from build123d import *

# Parameters (mm, degrees)
BOSS_EXTRUDE1_DEPTH = 1.524


with BuildPart() as part:
    # Sketch1 → Boss-Extrude1 (new body)
    with BuildSketch(Plane(origin=(0, 0, 0), x_dir=(1, 0, 0), z_dir=(0, 1, 0))):
        with BuildLine():
            Line((5.520593562, 10.562997869), (7.050708645, 17.571208446))
            ThreePointArc((7.050708645, 17.571208446), (7.131145016, 17.829150642), (7.238606677, 18.077054207))
            ThreePointArc((7.238606677, 18.077054207), (7.564510049, 19.45989002), (7.637457251, 20.878736946))
            ThreePointArc((7.637457251, 20.878736946), (8.492098945, 20.073618252), (9.504942938, 19.47966911))
            ThreePointArc((9.504942938, 19.47966911), (10.499295157, 19.276273595), (11.333912028, 18.698761041))
            Line((11.333912028, 18.698761041), (10.277523058, 13.457219083))
            Line((10.277523058, 13.457219083), (11.773700319, 13.155201971))
            Line((11.773700319, 13.155201971), (12.828772876, 18.399768932))
            ThreePointArc((12.828772876, 18.399768932), (13.409499296, 18.538098505), (14.004660893, 18.584584187))
            ThreePointArc((14.004660893, 18.584584187), (16.746835107, 19.097796263), (19.463914435, 19.730556864))
            ThreePointArc((19.463914435, 19.730556864), (18.823035781, 17.184750652), (17.837865312, 14.751379768))
            ThreePointArc((17.837865312, 14.751379768), (17.528924841, 13.243726046), (16.651902084, 11.979093671))
            Line((16.651902084, 11.979093671), (13.544076564, 9.012401066))
            Line((13.544076564, 9.012401066), (14.59914963, 7.908648182))
            Line((14.59914963, 7.908648182), (17.221929817, 10.411217166))
            ThreePointArc((17.221929817, 10.411217166), (19.571015538, 11.015907736), (21.993615768, 10.893995741))
            ThreePointArc((21.993615768, 10.893995741), (20.058776223, 8.670441452), (18.698609679, 6.055533286))
            ThreePointArc((18.698609679, 6.055533286), (16.478620051, 2.831263642), (16.457225541, -1.083300314))
            ThreePointArc((16.457225541, -1.083300314), (16.55614989, -1.524335384), (16.589363804, -1.975106719))
            ThreePointArc((16.589363804, -1.975106719), (16.624442109, -4.753141238), (17.243254302, -7.461605332))
            ThreePointArc((17.243254302, -7.461605332), (15.84253831, -5.968117791), (14.035036599, -5.006115769))
            Line((14.035036599, -5.006115769), (12.161156101, -1.197565278))
            Line((12.161156101, -1.197565278), (10.792144449, -1.871143044))
            Line((10.792144449, -1.871143044), (12.582390495, -5.515217687))
            ThreePointArc((12.582390495, -5.515217687), (12.984657899, -6.771031753), (13.401445653, -8.022101696))
            ThreePointArc((13.401445653, -8.022101696), (10.284977839, -6.689966631), (7.846889336, -4.335676947))
            ThreePointArc((7.846889336, -4.335676947), (6.119650246, -3.528046665), (4.880261331, -4.977024464))
            Line((4.880261331, -4.977024464), (4.878620901, -9.02232865))
            ThreePointArc((4.878620901, -9.02232865), (3.451641907, -14.873313942), (2.99866015, -20.878736946))
            ThreePointArc((2.99866015, -20.878736946), (2.023183201, -17.933730156), (0.761997186, -15.099293685))
            Line((0.761997186, -15.099293685), (0.761997186, -7.081931903))
            Line((0.761997186, -7.081931903), (-0.761997186, -7.081931903))
            Line((-0.761997186, -7.081931903), (-0.761997186, -15.100287099))
            ThreePointArc((-0.761997186, -15.100287099), (-2.023137189, -17.934235169), (-2.99866015, -20.878736946))
            ThreePointArc((-2.99866015, -20.878736946), (-3.451641907, -14.873313942), (-4.878620901, -9.02232865))
            Line((-4.878620901, -9.02232865), (-4.880261331, -4.977024464))
            ThreePointArc((-4.880261331, -4.977024464), (-6.119650246, -3.528046665), (-7.846889336, -4.335676947))
            ThreePointArc((-7.846889336, -4.335676947), (-10.284977839, -6.689966631), (-13.401445653, -8.022101696))
            ThreePointArc((-13.401445653, -8.022101696), (-12.984657899, -6.771031753), (-12.582390495, -5.515217687))
            Line((-12.582390495, -5.515217687), (-10.792144449, -1.871143044))
            Line((-10.792144449, -1.871143044), (-12.161156101, -1.197565278))
            Line((-12.161156101, -1.197565278), (-14.035036599, -5.006115769))
            ThreePointArc((-14.035036599, -5.006115769), (-15.84253831, -5.968117791), (-17.243254302, -7.461605332))
            ThreePointArc((-17.243254302, -7.461605332), (-16.624442109, -4.753141238), (-16.589363804, -1.975106719))
            ThreePointArc((-16.589363804, -1.975106719), (-16.55614989, -1.524335384), (-16.457225541, -1.083300314))
            ThreePointArc((-16.457225541, -1.083300314), (-16.478620051, 2.831263642), (-18.698609679, 6.055533286))
            ThreePointArc((-18.698609679, 6.055533286), (-20.058776223, 8.670441452), (-21.993615768, 10.893995741))
            ThreePointArc((-21.993615768, 10.893995741), (-19.571015538, 11.015907736), (-17.221929817, 10.411217166))
            Line((-17.221929817, 10.411217166), (-14.59914963, 7.908648182))
            Line((-14.59914963, 7.908648182), (-13.544076564, 9.012401066))
            Line((-13.544076564, 9.012401066), (-16.651902084, 11.979093671))
            ThreePointArc((-16.651902084, 11.979093671), (-17.528924841, 13.243726046), (-17.837865312, 14.751379768))
            ThreePointArc((-17.837865312, 14.751379768), (-18.823035781, 17.184750652), (-19.463914435, 19.730556864))
            ThreePointArc((-19.463914435, 19.730556864), (-16.746835107, 19.097796263), (-14.004660893, 18.584584187))
            ThreePointArc((-14.004660893, 18.584584187), (-13.409499296, 18.538098505), (-12.828772876, 18.399768932))
            Line((-12.828772876, 18.399768932), (-11.773700319, 13.155201971))
            Line((-11.773700319, 13.155201971), (-10.277523058, 13.457219083))
            Line((-10.277523058, 13.457219083), (-11.333912028, 18.698761041))
            ThreePointArc((-11.333912028, 18.698761041), (-10.499295157, 19.276273595), (-9.504942938, 19.47966911))
            ThreePointArc((-9.504942938, 19.47966911), (-8.492098945, 20.073618252), (-7.637457251, 20.878736946))
            ThreePointArc((-7.637457251, 20.878736946), (-7.564510049, 19.45989002), (-7.238606677, 18.077054207))
            ThreePointArc((-7.238606677, 18.077054207), (-7.131145016, 17.829150642), (-7.050708645, 17.571208446))
            Line((-7.050708645, 17.571208446), (-5.520593562, 10.562997869))
            ThreePointArc((-5.520593562, 10.562997869), (-3.516439493, 7.545594261), (0.000595641, 6.678517605))
            ThreePointArc((0.000595641, 6.678517605), (3.516886937, 7.546036839), (5.520593562, 10.562997869))
        make_face()
    extrude(amount=BOSS_EXTRUDE1_DEPTH)


solid = part.part
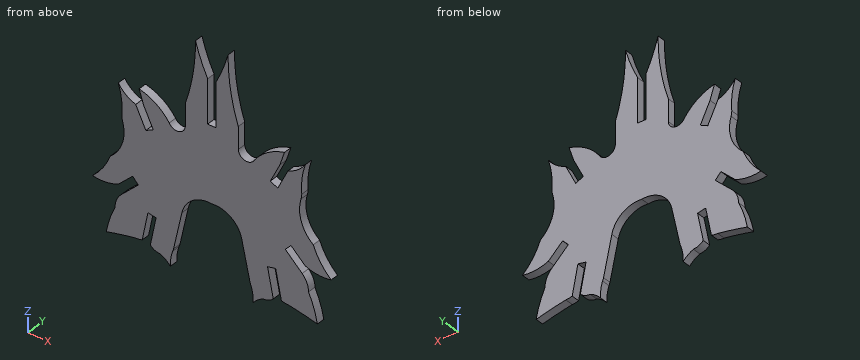
Part model, mm, in its own coordinate system. Coordinates: 2 decimals unless noted, no trailing zeros. Order: outer loops, then holes, each group sorted by start corner. A loop starts at its lowest first (then second) coordinate and runs counter-clockwise, first axis right, second up. Notation, with made-up numbers: M 24.5,-11 L 53.5,-11 A26 ccw 53.5,6 Z; hole C 47,-8 d9. An arc over 180 degrees is marked long. One line per question, with ' | ' between items.
Q1. Slice it at C-C (x = 3.5). Give the cut face in (y, z), and give its area (3 significant figures).
A:
outline: M 0,-7.53 L 1.52,-7.53 L 1.52,14.58 L 0,14.58 Z | area: 33.7 mm^2
Q2. Slice it at A-A (z = -14). Give the cut face in (x, y), and give its area (3 significant figures).
A:
outline: M -17.76,0 L -11.94,0 L -11.94,1.52 L -17.76,1.52 Z; M -10.39,0 L -6.27,0 L -6.27,1.52 L -10.39,1.52 Z; M 6.27,0 L 10.39,0 L 10.39,1.52 L 6.27,1.52 Z; M 11.94,0 L 17.76,0 L 17.76,1.52 L 11.94,1.52 Z | area: 30.3 mm^2
Q3. Drill centre lines: line 1 (X direction, y = 1.15, z = -16); line 2 (X direction, y = 0.7, z = -15); line 3 (Z direction, x = -14, y = 0.75). Where is each one in solid material? Low to high.
A:
line 1: x = -18.39 to -12.35, -10.79 to -6.71, 6.71 to 10.79, 12.35 to 18.39 | line 2: x = -17.96 to -12.14, -10.59 to -6.49, 6.49 to 10.59, 12.14 to 17.96 | line 3: z = -18.58 to -9.45, -8.54 to 4.93
Q4. Slice it at B-B (z = -4.5). Give the cut face in (x, y).
A:
outline: M -17.27,0 L 17.27,0 L 17.27,1.52 L -17.27,1.52 Z
Q5. Pin check, flat tips, straight feed: P1, Ø0.5, axis at y = 0.5, z = 9.5, coming from the -X side; P2, Ø0.5, axis at x = 0, y = 0.5, coming from the +Z side. Stop position of each tip, or through.
A:
P1: stops at x = -4.8 | P2: stops at z = 7.08
